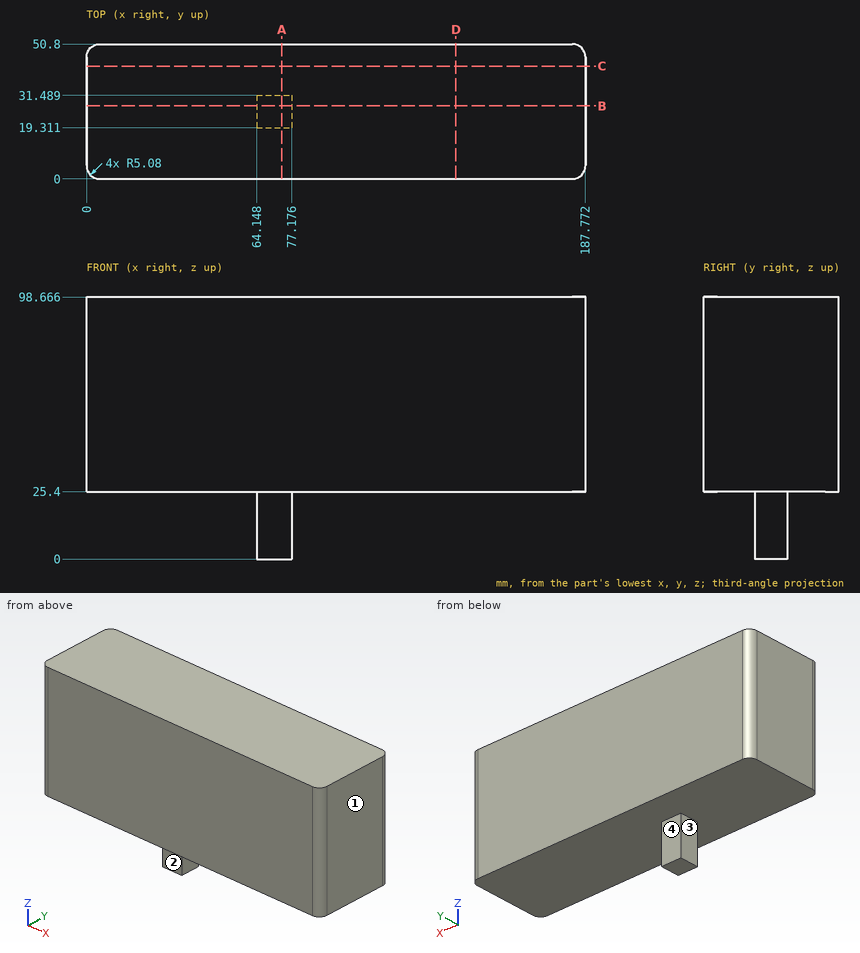
Here's the drawing with two shaded views (mm, measured from the low corner). I have some questions. A direction names the side the tool comes from. Round coordinates to 2 decimals unless told otherwise and drop trailing zeros. Loops run counter-clockwise (first coordinate to the right, second up) from the corner with the lowest first, then second, coordinate; pieces in that order, holes last.
1. Suppose I cut it at B-B, the plane y = 27.5. Please give me the cut outline in (x, z), and give its area (3 significant figures).
Answers:
outline: (0, 25.4) - (64.15, 25.4) - (64.15, 0) - (77.18, 0) - (77.18, 25.4) - (187.77, 25.4) - (187.77, 98.67) - (0, 98.67) - close
area: 14,100 mm2
2. Suppose I cut it at D-D, the plane x = 139. Please give me the cut outline in (y, z).
Answers:
outline: (0, 25.4) - (50.8, 25.4) - (50.8, 98.67) - (0, 98.67) - close
3. Suppose I cut it at C-C, the plane y = 42.5. Please give me the cut outline in (x, z), and give its area (3 significant figures).
Answers:
outline: (0, 25.4) - (187.77, 25.4) - (187.77, 98.67) - (0, 98.67) - close
area: 13,800 mm2
4. Will these pins go through, and if not, where does the flat tip stop? pin 1 (4 mm diameter, centred on x = 72.5, z = 9, fed in from -Y); pin 2 (12 mm diameter, centred on y = 30, z = 19.5, fed in from +X); pin 3 (3.5 mm diameter, centred on y = 24, z = 16.5, fed in from -X); pin 4 (9.5 mm diameter, centred on y = 28.5, z = 12, fed in from +X).
Answers:
pin 1: stops at y = 19.31
pin 2: stops at x = 187.77
pin 3: stops at x = 64.15
pin 4: stops at x = 77.18
5. For the marked faces 1, 2, 3 and 4, which set-ups out of +Z, -Z, +X, -X, +Y, -Y let a thin tool reach every point of the face, with its end or its side?
Answers:
face 1: +Z, -Z, +X, +Y, -Y
face 2: -Z, +X, -X, -Y
face 3: -Z, -X, +Y, -Y
face 4: -Z, +X, -X, +Y
6. If I drill on probe 1 along Z at (x, y) = (17.5, 28.5); probe 2 along X at (y, z) = (21, 10), over which ranges is the centre line in solid material (lowest first)?
Answers:
probe 1: z = 25.4 to 98.67
probe 2: x = 64.15 to 77.18
7. Suppose I cut it at A-A, the plane x = 73.5. Please give me the cut outline in (y, z), and give its area (3 significant figures).
Answers:
outline: (0, 25.4) - (19.31, 25.4) - (19.31, 0) - (31.49, 0) - (31.49, 25.4) - (50.8, 25.4) - (50.8, 98.67) - (0, 98.67) - close
area: 4,030 mm2
